Geometry check sheet. Reference: the model listing, model coordinates, mm. A direction names the side the tool comes from. Round coordinates to 2 decimals unless told otherwise and drop trailing zeros. Order: outer loops, then holes, each group sorted by start corner. A loop starts at its lowest first (then second) coordinate and runs counter-clockwise, first axis right, second up. Notation, with made-up numbers: M 80.5,5.25 L 133.5,5.25 A28 cw 133.5,31.25 Z; hole C 83,84 d2. An arc over 180 degrees is marked long. Answer as a JSON object with one key per item and string values. Group by question number.
```python
from build123d import *

# Parameters (mm, degrees)
F0_R     = 100
F1_DEPTH = 250
F2_R     = 50
F3_W     = 150
F3_H     = 90
F4_DEPTH = 25


with BuildPart() as f1:
    # F0 (on Front) → F1 (new body)
    with BuildSketch(Plane.XZ):
        with BuildLine():
            Line((-327.409887, 864.442099), (-677.409887, 864.442099))
            ThreePointArc((-677.409887, 864.442099), (-854.186583, 791.218795), (-927.409887, 614.442099))
            Line((-927.409887, 614.442099), (-927.409887, 264.442099))
            ThreePointArc((-927.409887, 264.442099), (-883.475904, 158.376082), (-777.409887, 114.442099))
            Line((-777.409887, 114.442099), (-177.409887, 114.442099))
            ThreePointArc((-177.409887, 114.442099), (-0.633192, 187.665404), (72.590113, 364.442099))
            Line((72.590113, 364.442099), (72.590113, 464.442099))
            ThreePointArc((72.590113, 464.442099), (64.021935, 546.789705), (38.684472, 625.609466))
            Line((38.684472, 625.609466), (-128.117229, 452.820158))
            ThreePointArc((-128.117229, 452.820158), (-372.385207, 452.459405), (-364.855767, 696.611577))
            Line((-364.855767, 696.611577), (-202.457301, 844.424798))
            ThreePointArc((-202.457301, 844.424798), (-264.136984, 859.406072), (-327.409887, 864.442099))
        make_face()
        with Locations((-650.047123, 488.092989)):
            Circle(F0_R, mode=Mode.SUBTRACT)
    extrude(amount=F1_DEPTH)

    # F2
    f2_edges = [f1.edges().sort_by_distance(p)[0] for p in [
        (-502.409887, -250, 864.442099),
        (-502.409887, 0, 864.442099),
    ]]
    fillet(f2_edges, radius=F2_R)

    # F3 (on face) → F4 (cut)
    with BuildSketch(Plane(origin=(-292.586202, 0, 282.447316), x_dir=(0, -1, 0), z_dir=(-0.719463, 0, 0.694531))):
        with Locations((125, 431.970147)):
            Rectangle(F3_W, F3_H)
    extrude(amount=-F4_DEPTH, mode=Mode.SUBTRACT)


solid = f1.part
```
1) Sectioned sample at C-C (y = -165). Record the boundary of the cut face in (x, z), then the cut area to 3 significant figures.
2) Go/stop test with flat-tipped pins: P1, Ø3, axis at x = -784, y = -144.5, coming from the -Z side; P2, Ø1, axis at x = -643.5, y = -205.5, coming from the -Z side; P3, Ø6, axis at y = -216.5, z = 333, coming from the -X side. Record where each tip stops, or that it passes through.
3) Release check for a two-part mould opening along Z. For faces 1 (the flat face through (-534, -250, 422)), 2 (the cylindrical face through (-554.665, -123.25, 518.13)), 3 (the cylindrical face through (-2.59, -123.95, 185.73)) record: +Z half, -Z half, draft (parallel to the pull), parting line (faces both ways), or undercut.
4) Sectioned sample at B-B (x = -390.5). Record the boundary of the cut face in (y, z), then the cut area to 3 significant figures.
5) Thickness scan on line 1 along X through (y, z) = (-122, 522); line 2 along X through (y, z) = (-105.5, 507); line 3 along Z through (x, y) = (-353.5, -77). Record the ranges inside material, lowest first. Write a range as [from, to].
6) Sectioned sample at A-A (z = 430). Record the boundary of the cut face in (x, y), then the cut area to 3 significant figures.
7) Set-up check for faces 4 (the flat face through (16, -200, 584)), 5 (the flat face through (-62.08, -123.25, 521.23)), 6 (the cylindrical face through (58.3, -235, 415.1)): record each of +Z, -Z, +X, -X, +Y, -Y from which the full face is reachable in a straight line by a thin tool's end or side.
Final values:
{
 "1": {"outline": "M -927.41,264.44 A150 ccw -777.41,114.44 L -177.41,114.44 A250 ccw 72.59,364.44 L 72.59,464.44 A400 ccw 48.86,600.16 L -5.84,543.49 L -23.82,560.86 L -128.12,452.82 A170 cw long -364.86,696.61 L -202.46,844.42 A400 ccw -327.41,864.44 L -677.41,864.44 A250 ccw -927.41,614.44 Z; hole C -650.05,488.09 d200", "area": "519,000 mm^2"},
 "2": {"P1": "stops at z = 114.53", "P2": "stops at z = 114.69", "P3": "stops at x = -925.55"},
 "3": {"face 1": "draft", "face 2": "undercut", "face 3": "-Z half"},
 "4": {"outline": "M -250,164.44 A50 ccw -200,114.44 L -50,114.44 A50 ccw 0,164.44 L 0,474.56 L -250,474.56 Z; M -250,667.22 L 0,667.22 L 0,814.44 A50 ccw -50,864.44 L -200,864.44 A50 ccw -250,814.44 Z", "area": "137,000 mm^2"},
 "5": {"line 1": "x = [-927.41, -744.12], [-555.97, -413.24], [-61.33, 68.43]", "line 2": "x = [-927.41, -748.24], [-551.85, -407.96], [-75.81, 70.32]", "line 3": "z = [114.44, 435.7], [706.95, 864.44]"},
 "6": {"outline": "M -927.41,-200 A50 ccw -877.41,-250 L -731.44,-250 L -731.44,0 L -877.41,0 A50 ccw -927.41,-50 Z; M -568.65,-250 L -345.56,-250 L -345.56,0 L -568.65,0 Z; M -155.3,-250 L 22.59,-250 A50 ccw 72.59,-200 L 72.59,-50 A50 ccw 22.59,0 L -155.3,0 Z", "area": "160,000 mm^2"},
 "7": {"face 4": "+Z", "face 5": "+Z, +Y, -Y", "face 6": "+Z, -Z, +X, -Y"}
}
